Autodesk Inventor part; units mm, degrees
ref_plane "YZ Plane" through (0, 0, 0) normal (1, 0, 0) x (0, 1, 0)
ref_plane "XZ Plane" through (0, 0, 0) normal (0, 1, 0) x (-1, 0, 0)
ref_plane "XY Plane" through (0, 0, 0) normal (0, 0, 1) x (1, 0, 0)
sketch "Sketch1" plane through (0, 0, 0) normal (0, 0, 1) x (1, 0, 0)
  arc A0 (-0.5, 10.6) -> (-2.5, 8.6) centre (-0.5, 8.6) ccw
  line L0 (-2.5, 8.6) -> (-2.5, -8.6)
  arc A1 (-2.5, -8.6) -> (-0.5, -10.6) centre (-0.5, -8.6) ccw
  line L1 (-0.5, -10.6) -> (2.5, -10.6)
  line L2 (2.5, -10.6) -> (2.5, 10.6)
  line L3 (2.5, 10.6) -> (-0.5, 10.6)
  line L4 (2.5, -51.8) -> (10.3, -51.8)
  arc A2 (10.3, -51.8) -> (12.3, -49.8) centre (10.3, -49.8) ccw
  line L5 (12.3, -49.8) -> (12.3, -43.8)
  arc A3 (14.3, -41.8) -> (12.3, -43.8) centre (14.3, -43.8) ccw
  line L6 (14.3, -41.8) -> (33.1, -41.8)
  arc A4 (35.1, -43.8) -> (33.1, -41.8) centre (33.1, -43.8) ccw
  line L7 (35.1, -43.8) -> (35.1, -49.8)
  arc A5 (35.1, -49.8) -> (37.1, -51.8) centre (37.1, -49.8) ccw
  line L8 (37.1, -51.8) -> (47.9, -51.8)
  arc A6 (47.9, -51.8) -> (49.9, -49.8) centre (47.9, -49.8) ccw
  line L9 (49.9, -49.8) -> (49.9, -27.6)
  arc A7 (51.9, -25.6) -> (49.9, -27.6) centre (51.9, -27.6) ccw
  line L10 (51.9, -25.6) -> (137.9, -25.6)
  arc A8 (139.9, -27.6) -> (137.9, -25.6) centre (137.9, -27.6) ccw
  line L11 (139.9, -27.6) -> (139.9, -49.8)
  arc A9 (139.9, -49.8) -> (141.9, -51.8) centre (141.9, -49.8) ccw
  line L12 (141.9, -51.8) -> (154.1, -51.8)
  arc A10 (154.1, -51.8) -> (156.1, -49.8) centre (154.1, -49.8) ccw
  line L13 (156.1, -49.8) -> (156.1, -41.8)
  line L14 (156.1, -41.8) -> (176.1, -41.8)
  line L15 (176.1, -41.8) -> (176.1, -49.8)
  arc A11 (176.1, -49.8) -> (178.1, -51.8) centre (178.1, -49.8) ccw
  line L16 (178.1, -51.8) -> (190.3, -51.8)
  arc A12 (190.3, -51.8) -> (192.3, -49.8) centre (190.3, -49.8) ccw
  line L17 (192.3, -49.8) -> (192.3, -38.8)
  arc A13 (192.3, -38.8) -> (190.3, -36.8) centre (190.3, -38.8) ccw
  line L18 (190.3, -36.8) -> (189.3, -36.8)
  arc A14 (187.3, -34.8) -> (189.3, -36.8) centre (189.3, -34.8) ccw
  line L19 (187.3, -34.8) -> (187.3, -6.4)
  arc A15 (189.3, -4.4) -> (187.3, -6.4) centre (189.3, -6.4) ccw
  line L20 (189.3, -4.4) -> (190.3, -4.4)
  arc A16 (190.3, -4.4) -> (192.3, -2.4) centre (190.3, -2.4) ccw
  line L21 (192.3, -2.4) -> (192.3, 8.6)
  arc A17 (192.3, 8.6) -> (190.3, 10.6) centre (190.3, 8.6) ccw
  line L22 (190.3, 10.6) -> (178.1, 10.6)
  arc A18 (178.1, 10.6) -> (176.1, 8.6) centre (178.1, 8.6) ccw
  line L23 (176.1, 8.6) -> (176.1, 2.6)
  arc A19 (174.1, 0.6) -> (176.1, 2.6) centre (174.1, 2.6) ccw
  line L24 (174.1, 0.6) -> (158.1, 0.6)
  arc A20 (156.1, 2.6) -> (158.1, 0.6) centre (158.1, 2.6) ccw
  line L25 (156.1, 2.6) -> (156.1, 8.6)
  arc A21 (156.1, 8.6) -> (154.1, 10.6) centre (154.1, 8.6) ccw
  line L26 (154.1, 10.6) -> (141.9, 10.6)
  arc A22 (141.9, 10.6) -> (139.9, 8.6) centre (141.9, 8.6) ccw
  line L27 (139.9, 8.6) -> (139.9, -13.6)
  arc A23 (137.9, -15.6) -> (139.9, -13.6) centre (137.9, -13.6) ccw
  line L28 (51.9, -15.6) -> (137.9, -15.6)
  arc A24 (49.9, -13.6) -> (51.9, -15.6) centre (51.9, -13.6) ccw
  line L29 (49.9, -13.6) -> (49.9, 8.6)
  arc A25 (49.9, 8.6) -> (47.9, 10.6) centre (47.9, 8.6) ccw
  line L30 (47.9, 10.6) -> (37.1745, 10.6)
  arc A26 (37.1745, 10.6) -> (35.1745, 8.6) centre (37.1745, 8.6) ccw
  line L31 (35.1745, 8.6) -> (35.1745, 2.6)
  arc A27 (33.1745, 0.6) -> (35.1745, 2.6) centre (33.1745, 2.6) ccw
  line L32 (33.1745, 0.6) -> (14.3, 0.6)
  arc A28 (12.3, 2.6) -> (14.3, 0.6) centre (14.3, 2.6) ccw
  line L33 (12.3, 2.6) -> (12.3, 8.6)
  arc A29 (12.3, 8.6) -> (10.3, 10.6) centre (10.3, 8.6) ccw
  line L34 (10.3, 10.6) -> (2.5, 10.6)
  line L35 (2.5, 10.6) -> (2.5, -51.8)
  circle A30 centre (181.65, 5.6) radius 1.25
  circle A31 centre (181.65, -46.8) radius 1.25
  circle A32 centre (150.55, -46.8) radius 1.25
  circle A33 centre (166.1, -20.6) radius 12.5
  circle A34 centre (150.55, 5.6) radius 1.25
  circle A35 centre (39.25, -46.8) radius 1.25
  circle A36 centre (8.15, 5.6) radius 1.25
  circle A37 centre (8.15, -46.8) radius 1.25
  circle A38 centre (23.7, -20.6) radius 12.5
  circle A39 centre (39.25, 5.6) radius 1.25
  arc A40 (-0.5, -30.6) -> (-2.5, -32.6) centre (-0.5, -32.6) ccw
  line L36 (-2.5, -32.6) -> (-2.5, -49.8)
  arc A41 (-2.5, -49.8) -> (-0.5, -51.8) centre (-0.5, -49.8) ccw
  line L37 (-0.5, -51.8) -> (2.5, -51.8)
  line L38 (2.5, -51.8) -> (2.5, -30.6)
  line L39 (2.5, -30.6) -> (-0.5, -30.6)
  arc A42 (-0.5, 12.6) -> (-4.5, 8.6) centre (-0.5, 8.6) ccw
  line L40 (-4.5, 8.6) -> (-4.5, -8.6)
  arc A43 (-4.5, -8.6) -> (-0.5, -12.6) centre (-0.5, -8.6) ccw
  line L41 (-0.5, -12.6) -> (4.5, -12.6)
  line L42 (4.5, -12.6) -> (4.5, 12.6)
  line L43 (4.5, 12.6) -> (-0.5, 12.6)
  arc A44 (-0.5, -28.6) -> (-4.5, -32.6) centre (-0.5, -32.6) ccw
  line L44 (-0.5, -28.6) -> (4.5, -28.6)
  line L45 (4.5, -28.6) -> (4.5, -53.8)
  line L46 (4.5, -53.8) -> (-0.5, -53.8)
  arc A45 (-4.5, -49.8) -> (-0.5, -53.8) centre (-0.5, -49.8) ccw
  line L47 (-4.5, -49.8) -> (-4.5, -32.6)
  line L48 (4.5, -12.6) -> (4.5, -28.6)
  line L49 (-4.5, -8.6) -> (-4.5, -32.6)
  line L50 (0, -28.6) -> (0, -12.6)
  line L51 (-3, -12.6) -> (3, -12.6)
  line L52 (3, -12.6) -> (3, -28.6)
  line L53 (3, -28.6) -> (-3, -28.6)
  line L54 (-3, -28.6) -> (-3, -12.6)
  line L55 (-3, -12.6) -> (3, -28.6) construction
  line L56 (3, -12.6) -> (-3, -28.6) construction
  arc A46 (-0.5, -30.5065) -> (-2.5935, -32.6) centre (-0.5, -32.6) ccw
  line L57 (-0.5, -30.5065) -> (2.5935, -30.5065)
  line L58 (2.5935, -30.5065) -> (2.5935, -51.8935)
  line L59 (2.5935, -51.8935) -> (-0.5, -51.8935)
  arc A47 (-2.5935, -49.8) -> (-0.5, -51.8935) centre (-0.5, -49.8) ccw
  line L60 (-2.5935, -49.8) -> (-2.5935, -32.6)
  arc A48 (-2.6, -8.6) -> (-0.5, -10.7) centre (-0.5, -8.6) ccw
  line L61 (-2.6, -8.6) -> (-2.6, 8.6)
  arc A49 (-0.5, 10.7) -> (-2.6, 8.6) centre (-0.5, 8.6) ccw
  line L62 (-0.5, 10.7) -> (2.6, 10.7)
  line L63 (2.6, 10.7) -> (2.6, -10.7)
  line L64 (2.6, -10.7) -> (-0.5, -10.7)
  line L65 (2.5, -12.6) -> (2.5, -13.431)
  line L66 (2.5, -13.431) -> (2.5, -15.7904)
  line L67 (2.5, -15.7904) -> (2.5, -28.2258)
  line L68 (2.5, -28.2258) -> (2.5, -28.5718)
  line L69 (2.5, -28.5718) -> (2.5, -28.6211)
  line L70 (4.5, 12.6) -> (-4.5, 12.6)
  line L71 (-4.5, 12.6) -> (-4.5, -53.8)
  line L72 (-4.5, -53.8) -> (4.5, -53.8)
  line L73 (4.5, -53.8) -> (4.5, 12.6)
  point P0 (0, 0)
  point P1 (0, -20.6)
  point P2 (2.5, -12.6)
  point P3 (2.5, -28.6)
  point P4 (2.5935, -51.8)
  point P5 (4.5, -51.8)
  point P6 (2.5, -30.5065)
  point P7 (-0.5, -28.6)
  point P8 (-0.5, -12.6)
  point P9 (2.5, -10.7)
  point P10 (4.5, 10.6)
  point P11 (2.6, 10.6)
  point P12 (-4.5, 8.6)
  point P13 (-0.5, 12.6)
  point P14 (-0.5, -53.8)
  point P15 (-4.5, -49.8)
  dimension "d0" = 2
  dimension "d1" = 2
  dimension "d2" = 6
  dimension "d3" = 0.1
extrude "Extrusion1" add sketch "Sketch1" along normal blind 10 contours L63 L62 A49 L61 A48 L64 L35 L41 A43 L40 A42 L43 L42 L34 | L34 L42 L41 L35 L64 L63 | L41 L52 L44 L35 | L48 L44 L52 L41 | L45 L4 L58 L57 L35 L44 | A42 L71 L70 | L51 L54 L53 A44 L49 A43 | L44 L35 L57 A46 L60 A47 L59 L58 L4 L45 L46 A45 L47 A44 | L72 L71 A45
sketch "Sketch10" plane through (-4.5, -53.8, 0) normal (-1, 0, 0) x (0, 0, 1)
  line L0 (0, 66.4) -> (0, 0)
  line L1 (0, 0) -> (10, 0)
  line L2 (10, 66.4) -> (10, 0)
  line L3 (0, 66.4) -> (10, 66.4)
  line L4 (0, 1.9065) -> (0, 0)
  line L5 (0, -7.3) -> (10, -7.3)
  line L6 (10, -7.3) -> (10, 73.7)
  line L7 (10, 73.7) -> (0, 73.7)
  line L8 (0, 73.7) -> (10, -7.3) construction
  line L9 (0, -7.3) -> (10, 73.7) construction
  line L10 (0, 1.9065) -> (10, 1.9065)
  line L11 (0, 73.7) -> (81, 73.7) construction
  line L12 (12, -9.3) -> (-2, -9.3)
  line L13 (-2, -9.3) -> (-2, 75.7)
  line L14 (-2, 75.7) -> (12, 75.7)
  line L15 (12, 75.7) -> (12, -9.3)
  line L16 (0, 73.7) -> (-40, 73.7)
  line L17 (-40, 73.7) -> (-40, -7.3)
  line L18 (-40, -7.3) -> (0, -7.3)
  line L19 (0, 0) -> (0, 1.9065)
  line L20 (-42, 75.7) -> (2, 75.7)
  line L21 (2, -9.3) -> (-42, -9.3)
  line L22 (-42, -9.3) -> (-42, 75.7)
  line L23 (2, -7.3) -> (2, -9.3)
  line L24 (10, -7.3) -> (10, -9.3)
  line L25 (10, 73.7) -> (10, 75.7)
  point P0 (0, 53.8)
  point P1 (5, 33.2)
  point P2 (-2, -9.3)
  point P3 (-2, 73.7)
  point P4 (-2, -9.3)
  point P5 (-2, -7.3)
  dimension "d64" = 81
  dimension "d65" = 90
  dimension "d66" = 2
  dimension "d67" = 40
  dimension "d68" = 2
extrude "Extrusion9" add sketch "Sketch10" along normal blind 2
extrude "Extrusion10" add sketch "Sketch10" along normal blind 30 contours L16 L17 L18 L13 L21 L22 L20
properties part number "drzalo_vezja"
Build history of the part. All positions in model axes, mm. A direction names the side the tool comes from. Round coordinates to 2 decimals unless told otherwise and drop trailing zeros. Order: outer loops, then holes, each group sorted by start corner. A loop starts at its lowest first (then second) coordinate and runs counter-clockwise, first axis right, second up. Notation, with made-up numbers: M -20,12.5 L 16,12.5 A22 cw 16,19.5 Z; hole C 18.25,-23.75 d2. An arc over 180 degrees is marked long. Use CSV: the item, a comma, the result in double quotes. Start each with the question number.
(1) Cut at C-C on x = 1.5. List the corners of the cut face in (y, z).
(2) Cut at B-B on z = 7.5. List the corners of the cut face in (x, y).
(3) Tool access for faces 3 (the face through (-20, 19.9, -21)), 4 (the face through (-2.594, -41, 5)), 5 (the face through (-19, -63.1, -21)), 6 (the face through (3, -20, 10)), 7 (the face through (-20, 21, -2)): list every direction of +Z, -Z, +X, -X, +Y, -Y with a clear straight run to the whole face (end or side of a thin tool).
(4) Flat gauge pins, fed straight in: P1, Ø4.5, axis at x = 1.5, y = -29, coming from the -Z side; P2, Ø15.5, axis at y = -13.5, z = -7, coming from the -X side; P3, Ø10, axis at x = 1, y = -25, coming from the +Z side. Where does each tip first touch, or does it go through?
(5) Cut at A-A on y = -22. List the corners of the cut face in (x, z), then the cut area to 3 significant figures.
(6) Drill centre lines: probe 1 along Y at (x, z) = (0, 6); probe 2 along Y at (x, z) = (-30.5, -24); probe 3 along Z at (x, y) = (-22.5, -15). Where is each one in solid material? Low to high.
(7) Mould opens along X. For faces 1 (the face through (-2.6, 0, 5)), 2 (the face through (0, 12.6, 5)) say: +X half, -X half, draft (parallel to the pull), parting line (faces both ways), or undercut.
(8) Cut at D-D on x = -20. List the corners of the cut face in (y, z), then the cut area to 3 significant figures.
Findings:
1,outline,"M -53.8,0 L -51.89,0 L -51.89,10 L -53.8,10 Z; M -30.51,0 L -28.6,0 L -28.6,10 L -30.51,10 Z; M -12.6,0 L -10.7,0 L -10.7,10 L -12.6,10 Z; M 10.7,0 L 12.6,0 L 12.6,10 L 10.7,10 Z"
2,outline,"M -6.5,-63.1 L -4.5,-63.1 L -4.5,-53.8 L 4.5,-53.8 L 4.5,12.6 L -4.5,12.6 L -4.5,21.9 L -6.5,21.9 Z; hole M -3,-28.6 L 2.5,-28.6 L 2.5,-12.6 L -3,-12.6 Z; hole M -2.6,-8.6 A2.1 ccw -0.5,-10.7 L 2.6,-10.7 L 2.6,10.7 L -0.5,10.7 A2.1 ccw -2.6,8.6 Z; hole M -2.59,-49.8 A2.09 ccw -0.5,-51.89 L 2.59,-51.89 L 2.59,-30.51 L -0.5,-30.51 A2.09 ccw -2.59,-32.6 Z"
3,face 3,"+Z, -X"
3,face 4,"+Z, -Z"
3,face 5,"+Z, -Z, +X, -X, -Y"
3,face 6,"+Z, +X, +Y, -Y"
3,face 7,"+Z, -X, +Y, -Y"
4,P1,"stops at z = 0"
4,P2,"stops at x = -6.5"
4,P3,"stops at z = 10"
5,outline,"M -34.5,-42 L -4.5,-42 L -4.5,0 L -3,0 L -3,10 L -4.5,10 L -4.5,12 L -6.5,12 L -6.5,-40 L -34.5,-40 Z; M 2.5,0 L 4.5,0 L 4.5,10 L 2.5,10 Z"
5,area,"199 mm^2"
6,probe 1,"y = -53.8 to -51.89, -30.51 to -28.6, -12.6 to -10.7, 10.7 to 12.6"
6,probe 2,"y = -63.1 to -61.1, 19.9 to 21.9"
6,probe 3,"z = -42 to -40"
7,face 1,"undercut"
7,face 2,"draft"
8,outline,"M -63.1,-42 L 21.9,-42 L 21.9,-2 L 19.9,-2 L 19.9,-40 L -61.1,-40 L -61.1,-2 L -63.1,-2 Z"
8,area,"322 mm^2"
